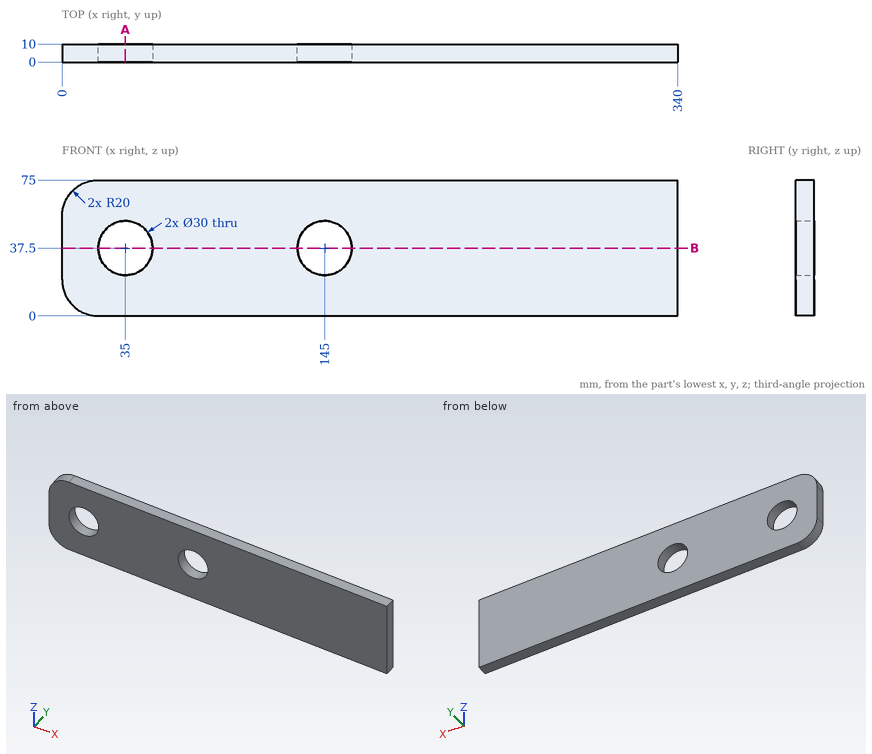
Can you work these out from the drawing? Everything is in mm from the part's minimum corner. Give positions to 0.01 mm unless a question says otherwise; leave off trailing zeros. Order: outer loops, then holes, each group sorted by start corner. A loop starts at its lowest first (then second) coordinate and runs counter-clockwise, first axis right, second up.
1. Suppose I cut it at B-B (z = 37.5). List the corners of the cut face in (x, y) for me.
2. Suppose I cut it at A-A (x = 35). List the corners of the cut face in (y, z) for me, plus the area to 3 significant figures.
3. I need wall thicknesses on L1, parallel to X at y = 3.75, z = 37.5; L2, parallel to Z at x = 145, y = 6.75; L3, parallel to X at y = 1.5, z = 25. Which ranges of each line are inside material? Lowest first, please.
4. Will this pin go through, and if not, where does the flat tip stop? P1, Ø24, axis at x = 145, z = 37.5, coming from the +Y side.
Solved:
1. outline: (0, 0) - (20, 0) - (20, 10) - (0, 10) - close; (50, 0) - (130, 0) - (130, 10) - (50, 10) - close; (160, 0) - (340, 0) - (340, 10) - (160, 10) - close
2. outline: (0, 0) - (10, 0) - (10, 22.5) - (0, 22.5) - close; (0, 52.5) - (10, 52.5) - (10, 75) - (0, 75) - close
2. area: 450 mm2
3. L1: x = 0 to 20, 50 to 130, 160 to 340
3. L2: z = 0 to 22.5, 52.5 to 75
3. L3: x = 0 to 26.71, 43.29 to 136.71, 153.29 to 340
4. P1: passes through
